Geometry: final body of the model. Coordinates: model frame, mm. Coordinates: 2 decimals unless noted, no trailing zeros. Write each loop counter-clockwise with the first axis right and the second up, starting at its lowest first coordinate (ties: lowest second). Pieces come first, ordered by that corner, then holes. Notation, with made-up numbers: (34, -34) - (60, -34) arc R26 ccw to (60, 5) - close; hole circle Ø7 at (85.25, 56.5). An arc over 180 degrees is marked (long way). Answer as a JSON object with one key per item and string values. Group by question number.
Item 1: Section A-A on z = 0. Return loops of the section in (x, y) (3 decimals).
Item 2: Section B-B on x = 28.5. Return loops of the section in (y, z) (3 decimals), and give its area (3 significant figures).
Item 3: Line query: line 1 along Z through (x, y) = (-172, 4.75); line 2 along Z through (x, y) = (80.91, 4); line 3 along Z through (x, y) = (94, 4). Output: solid intervals per line, ascending. Write a range as from..to.
```python
from build123d import *

# Parameters (mm, degrees)
SKETCH1_W                         = 407
SKETCH1_H                         = 122
BASE_PLATE_DEPTH                  = 6.35
SKETCH2_R                         = 2.675
IGBT_HOLES_DEPTH                  = 7.35
IGBT_HOLES_PATTERN_COUNT          = 3
IGBT_HOLES_PATTERN_PITCH          = 66.5
IGBT_HOLES_MIRROR_COPY_1_SKETCH_R = 2.675
IGBT_HOLES_MIRROR_COPY_1_DEPTH    = 7.35
IGBT_HOLES_MIRROR_COPY_2_SKETCH_R = 2.675
IGBT_HOLES_MIRROR_COPY_2_DEPTH    = 7.35


with BuildPart() as part:
    # Sketch1 → Base Plate (new body)
    with BuildSketch(Plane(origin=(0, 0, 0), x_dir=(1, 0, 0), z_dir=(0, 1, 0))):
        Rectangle(SKETCH1_W, SKETCH1_H)
    extrude(amount=BASE_PLATE_DEPTH)

    # Sketch2 → IGBT Holes (cut, through all)
    with BuildSketch(Plane(origin=(0, 6.35, 0), x_dir=(1, 0, 0), z_dir=(0, 1, 0))):
        with Locations((197.595, 55.095)):
            Circle(SKETCH2_R)
        with Locations((197.595, -55.095)):
            Circle(SKETCH2_R)
        with Locations((147.41, -55.095)):
            Circle(SKETCH2_R)
        with Locations((147.41, 55.095)):
            Circle(SKETCH2_R)
    igbt_holes = extrude(amount=-IGBT_HOLES_DEPTH, mode=Mode.SUBTRACT)

    # IGBT Holes Pattern: IGBT Holes ×3
    with Locations(*[(-i * IGBT_HOLES_PATTERN_PITCH, 0, 0) for i in range(1, IGBT_HOLES_PATTERN_COUNT)]):
        add(igbt_holes, mode=Mode.SUBTRACT)

    # IGBT Holes Mirror: IGBT Holes across plane
    add(igbt_holes.mirror(Plane(origin=(0, 0, 0), x_dir=(0, 0, 1), z_dir=(1, 0, 0))), mode=Mode.SUBTRACT)

    # IGBT Holes Mirror copy 1 sketch → IGBT Holes Mirror copy 1 (cut, through all)
    with BuildSketch(Plane(origin=(66.5, 6.35, 0), x_dir=(-1, 0, 0), z_dir=(0, 1, 0))):
        with Locations((197.595, -55.095)):
            Circle(IGBT_HOLES_MIRROR_COPY_1_SKETCH_R)
        with Locations((197.595, 55.095)):
            Circle(IGBT_HOLES_MIRROR_COPY_1_SKETCH_R)
        with Locations((147.41, 55.095)):
            Circle(IGBT_HOLES_MIRROR_COPY_1_SKETCH_R)
        with Locations((147.41, -55.095)):
            Circle(IGBT_HOLES_MIRROR_COPY_1_SKETCH_R)
    extrude(amount=-IGBT_HOLES_MIRROR_COPY_1_DEPTH, mode=Mode.SUBTRACT)

    # IGBT Holes Mirror copy 2 sketch → IGBT Holes Mirror copy 2 (cut, through all)
    with BuildSketch(Plane(origin=(133, 6.35, 0), x_dir=(-1, 0, 0), z_dir=(0, 1, 0))):
        with Locations((197.595, -55.095)):
            Circle(IGBT_HOLES_MIRROR_COPY_2_SKETCH_R)
        with Locations((197.595, 55.095)):
            Circle(IGBT_HOLES_MIRROR_COPY_2_SKETCH_R)
        with Locations((147.41, 55.095)):
            Circle(IGBT_HOLES_MIRROR_COPY_2_SKETCH_R)
        with Locations((147.41, -55.095)):
            Circle(IGBT_HOLES_MIRROR_COPY_2_SKETCH_R)
    extrude(amount=-IGBT_HOLES_MIRROR_COPY_2_DEPTH, mode=Mode.SUBTRACT)

    # Pipe Profile: sweep along a path in Sketch3
    with BuildLine(Plane(origin=(0, 6.35, 0), x_dir=(1, 0, 0), z_dir=(0, 1, 0))) as pipe_profile_path:
        Line((-203.5, 25.4), (165.4, 25.4))
        ThreePointArc((165.4, 25.4), (190.8, 0), (165.4, -25.4))
        Line((165.4, -25.4), (-203.5, -25.4))
    # Sketch4 → Pipe Profile (sweep, cut)
    with BuildSketch(Plane.ZY.offset(203.5)):
        with BuildLine():
            Line((-28.575, 1.27), (-22.225, 1.27))
            ThreePointArc((-22.225, 1.27), (-19.97993597, 2.19993597), (-19.05, 4.445))
            Line((-19.05, 4.445), (-19.05, 6.35))
            Line((-19.05, 6.35), (-31.75, 6.35))
            Line((-31.75, 6.35), (-31.75, 4.445))
            ThreePointArc((-31.75, 4.445), (-30.82006403, 2.19993597), (-28.575, 1.27))
        make_face()
    sweep(path=pipe_profile_path.line, mode=Mode.SUBTRACT)


solid = part.part
```
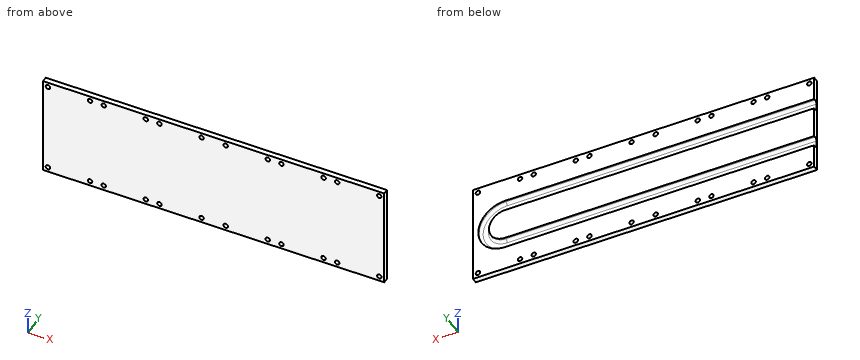
Checks:
{
 "1": {"outline": "(-203.5, 0) - (203.5, 0) - (203.5, 6.35) - (197.15, 6.35) - (197.15, 4.445) arc R3.175 cw to (193.975, 1.27) - (187.625, 1.27) arc R3.175 cw to (184.45, 4.445) - (184.45, 6.35) - (-203.5, 6.35) - close"},
 "2": {"outline": "(0, -61) - (6.35, -61) - (6.35, -31.75) - (4.445, -31.75) arc R3.175 cw to (1.27, -28.575) - (1.27, -22.225) arc R3.175 cw to (4.445, -19.05) - (6.35, -19.05) - (6.35, 19.05) - (4.445, 19.05) arc R3.175 cw to (1.27, 22.225) - (1.27, 28.575) arc R3.175 cw to (4.445, 31.75) - (6.35, 31.75) - (6.35, 61) - (0, 61) - close", "area": "654 mm^2"},
 "3": {"line 1": "-61..-31.75, -19.05..19.05, 31.75..61", "line 2": "-61..-57.77, -52.42..-31.72, -19.08..19.08, 31.72..52.42, 57.77..61", "line 3": "-61..-31.72, -19.08..19.08, 31.72..61"}
}
